Could you check a few things on this model? Use its own coordinates, in mm. A direction names the side the tool comes from. Give positions to 0.01 mm unless a question says otherwise; leave off trailing zeros. Loops run counter-clockwise (first coordinate to the right, second up) from the corner with the lowest first, then second, coordinate; pieces in that order, holes last. Notation, with made-up numbers: (-31.75, 23.25) -> (3.25, 23.25) arc R18 ccw to (3.25, 44.25) -> close; hole circle Ø4 at (89, -15). An arc over 180 degrees is marked (long way). Put each result on its own line as item: value.
```python
from build123d import *

# Parameters (mm, degrees)
F0_R     = 155.0189943433
F0_W     = 91.0461395979
F0_H     = 101.8910259008
F1_DEPTH = 50
F2_T     = -2.5
F3_DEPTH = 50
F4_DEPTH = 60


with BuildPart() as f1:
    # F0 (on Top) → F1 (new body)
    with BuildSketch(Plane.XY):
        Circle(F0_R)
        with Locations((45.5230697989, -5.9630684555)):
            Rectangle(F0_W, F0_H, mode=Mode.SUBTRACT)
    extrude(amount=F1_DEPTH)

    # F2
    f2_openings = [f1.faces().sort_by_distance(p)[0] for p in [
        (-6.37749, 0.835388, 50),
    ]]
    offset(amount=F2_T, openings=f2_openings, kind=Kind.INTERSECTION)

    # F0 (on Top) → F3 (join)
    with BuildSketch(Plane.XY):
        Circle(F0_R)
        with Locations((45.5230697989, -5.9630684555)):
            Rectangle(F0_W, F0_H, mode=Mode.SUBTRACT)
    extrude(amount=-F3_DEPTH)

    # F4 (add): a face of the model
    f4_faces = [f1.faces().sort_by_distance(p)[0] for p in [
        (-7.4404710718, 0.9746275578, 2.5),
    ]]
    extrude(f4_faces, amount=-F4_DEPTH)


solid = f1.part
```
1. Thinking about a two-plate mould opening in X: for faces 1 (the face through (145.476, -45.813, -53.698)), 2 (the face through (114, -103, 50)), 3 (the face through (-2.5, -7, 26)), which applies, pulls with the +X half, pulls with the -X half, needs draft (parallel to the pull), parting line crosses it, or undercut?
Recorded:
face 1: parting line crosses it
face 2: needs draft
face 3: undercut
2. If we section it at B-B (y = -4): List the corners of the cut face in (x, z) for me, then the cut area to 3 significant figures.
Recorded:
outline: (-154.97, -50) -> (-152.47, -50) -> (-152.47, -57.5) -> (-2.5, -57.5) -> (-2.5, -50) -> (0, -50) -> (0, 50) -> (-2.5, 50) -> (-2.5, 2.5) -> (-152.47, 2.5) -> (-152.47, 50) -> (-154.97, 50) -> close; (91.05, -50) -> (93.55, -50) -> (93.55, -57.5) -> (152.47, -57.5) -> (152.47, -50) -> (154.97, -50) -> (154.97, 50) -> (152.47, 50) -> (152.47, 2.5) -> (93.55, 2.5) -> (93.55, 50) -> (91.05, 50) -> close
area: 13,500 mm^2
3. For faces 4 (the face through (45, -59.409, 26)), 5 (the face through (45, -59.409, -54)), 6 (the face through (-36, 2, -57.5)), 7 (the face through (91.046, -7, 1)), which set-ups out of +Z, -Z, +X, -X, +Y, -Y let a thin tool reach every point of the face, with its end or its side?
Recorded:
face 4: +Z
face 5: -Z
face 6: -Z, +X, -X, +Y, -Y
face 7: +Z, -Z
4. If we section it at D-D (y = 123): List the corners of the cut face in (x, z) for me, then the cut area to 3 significant figures.
Recorded:
outline: (-94.35, -50) -> (-90.18, -50) -> (-90.18, -57.5) -> (90.18, -57.5) -> (90.18, -50) -> (94.35, -50) -> (94.35, 50) -> (90.18, 50) -> (90.18, 2.5) -> (-90.18, 2.5) -> (-90.18, 50) -> (-94.35, 50) -> close
area: 11,700 mm^2
5. If we section it at A-A (z = -2): List the corners of the cut face in (x, y) for me.
Recorded:
outline: circle Ø310.04 at (0, 0); hole (0, -56.91) -> (91.05, -56.91) -> (91.05, 44.98) -> (0, 44.98) -> close
6. I'm going to push flat-ended pins straight in: pin 1 (14 mm diameter, centred on y = 18, z = 15, fed in from +X); pin 2 (8 mm diameter, centred on y = -28, z = -54.5, fed in from -X); pin 3 (6 mm diameter, centred on x = 120.5, y = 62, fed in from +Z). Where does each tip first touch, or does it pass through?
Recorded:
pin 1: stops at x = 154.63
pin 2: stops at x = -150.62
pin 3: stops at z = 2.5
7. I need wall thicknesses on line 1 (Y direction, x = 91, z = 39.5); line 2 (X direction, y = -56, z = 28.5); line 3 (Z direction, x = -53.5, y = 100). Which ranges of each line are inside material? Lowest first, please.
Recorded:
line 1: y = -125.5 to -122.4, -59.41 to -56.91, 44.98 to 47.48, 122.4 to 125.5
line 2: x = -144.55 to -141.87, -2.5 to 0, 91.05 to 93.55, 141.87 to 144.55
line 3: z = -57.5 to 2.5
8. If we section it at C-C (x = 64.5): List the corners of the cut face in (y, z) for me, then the cut area to 3 significant figures.
Recorded:
outline: (-140.96, -50) -> (-138.21, -50) -> (-138.21, -57.5) -> (-59.41, -57.5) -> (-59.41, -50) -> (-56.91, -50) -> (-56.91, 50) -> (-59.41, 50) -> (-59.41, 2.5) -> (-138.21, 2.5) -> (-138.21, 50) -> (-140.96, 50) -> close; (44.98, -50) -> (47.48, -50) -> (47.48, -57.5) -> (138.21, -57.5) -> (138.21, -50) -> (140.96, -50) -> (140.96, 50) -> (138.21, 50) -> (138.21, 2.5) -> (47.48, 2.5) -> (47.48, 50) -> (44.98, 50) -> close
area: 11,200 mm^2
